Here's how the part is built. I have some questions about the finished solid (model axes, mm). A direction names the side the tool comes from. Coordinates: 2 decimals unless noted, no trailing zeros. Loops run counter-clockwise (first coordinate to the right, second up) from the corner with the lowest first, then second, coordinate; pieces in that order, holes last. Notation, with made-up numbers: M -5,31.25 L 54,31.25 A25 ccw 54,64.25 Z; hole C 31,54.5 d7. An arc over 180 degrees is marked long. Use CSV: the item, a comma, the result in double quotes. Start each with the question number.
Q1. Which directions (+Z, -Z, +X, -X, +Y, -Y) give clear straight access to the entire face, cutting with the end or side of a thin tool? Please do faces 4 (the cylindrical face through (-18.539, -3.905, -0.867)), 5 (the cylindrical face through (-14.985, 14.584, -0.66)).
Q2. Please list where these lines run through material, in increasing order: probe 1 along Z at (x, y) = (16, 0); probe 2 along X at (y, z) = (-18, 0). Write a range as [from, to].
Q3. For pin 1 Ø24 at (y, z) = (0, 0) entering from +X; pin 2 Ø1.5 at (y, z) = (-1, 7.5) entering from +X; pin 3 Ø7 at (x, z) = (0, 0) entering from -Y, each with a flat end and sliding along its axis, tell me the tip position at first contact or that it passes through.
Q4. If we section it at D-D (z = -11): Please give me the cut outline in (x, y).
Q5. If we section it at A-A (x = 0): Please give me the cut outline in (y, z), and give its area (3 significant figures).
Q6. If we section it at C-C (z = 0): Please give me the cut outline in (x, y).
Q7. If we mould it in two halves opening along Z, with no side actions, what happens to faces 1 (the cylindrical face through (-1.748, 18.859, -18.797)), 2 (the cylindrical face through (14.584, -14.643, 3.252)), 3 (the flat face through (-15.4, 20, -0.1))? For each: +Z half, -Z half, draft (parallel to the pull), parting line (faces both ways), or undercut.
from build123d import *

# Parameters (mm, degrees)
SKETCH1_W           = 40
SKETCH1_H           = 40
BOSS_EXTRUDE1_DEPTH = 20
FILLET1_R           = 4
SKETCH12_R          = 15
CUT_EXTRUDE2_DEPTH  = 20
SKETCH13_R          = 15
CUT_EXTRUDE3_DEPTH  = 20
SKETCH16_R          = 4
CUT_EXTRUDE6_DEPTH  = 20
SKETCH17_R          = 4
CUT_EXTRUDE7_DEPTH  = 20


with BuildPart() as part:
    # Sketch1 → Boss-Extrude1 (new body, symmetric)
    with BuildSketch(Plane(origin=(0, 0, 0), x_dir=(1, 0, 0), z_dir=(0, 1, 0))):
        Rectangle(SKETCH1_W, SKETCH1_H)
    extrude(amount=BOSS_EXTRUDE1_DEPTH, both=True)

    # Fillet1
    fillet1_edges = [part.edges().sort_by_distance(p)[0] for p in [
        (20, 20, 0),
        (0, 20, -20),
        (20, 0, -20),
        (20, 0, 20),
        (0, 20, 20),
    ]]
    fillet(fillet1_edges, radius=FILLET1_R)

    # Sketch2 → Cut-Revolve1 (revolve, cut)
    with BuildSketch(Plane(origin=(0, 0, 0), x_dir=(1, 0, 0), z_dir=(0, 1, 0))):
        with BuildLine():
            Line((0, 17.5), (0, -17.5))
            ThreePointArc((0, -17.5), (-17.5, 0), (0, 17.5))
        make_face()
    revolve(axis=Axis((0, 0, -20.989422068), (0, 0, 1)), mode=Mode.SUBTRACT)

    # Sketch12 → Cut-Extrude2 (cut)
    with BuildSketch(Plane(origin=(0, 20, 0), x_dir=(1, 0, 0), z_dir=(0, 1, 0))):
        Circle(SKETCH12_R)
    extrude(amount=-CUT_EXTRUDE2_DEPTH, mode=Mode.SUBTRACT)

    # Sketch13 → Cut-Extrude3 (cut)
    with BuildSketch(Plane(origin=(20, 0, 0), x_dir=(0, 0, -1), z_dir=(1, 0, 0))):
        Circle(SKETCH13_R)
    extrude(amount=-CUT_EXTRUDE3_DEPTH, mode=Mode.SUBTRACT)

    # Sketch16 → Cut-Extrude6 (cut)
    with BuildSketch(Plane.XZ.offset(20)):
        Circle(SKETCH16_R)
    extrude(amount=-CUT_EXTRUDE6_DEPTH, mode=Mode.SUBTRACT)

    # Sketch17 → Cut-Extrude7 (cut)
    with BuildSketch(Plane.ZY.offset(20)):
        Circle(SKETCH17_R)
    extrude(amount=-CUT_EXTRUDE7_DEPTH, mode=Mode.SUBTRACT)


solid = part.part
Results below:
1,face 4,"+X, -X"
1,face 5,"+Y"
2,probe 1,"[-20, -15], [15, 20]"
2,probe 2,"[-20, -4], [4, 20]"
3,pin 1,"x = -12.74"
3,pin 2,"x = -15.4"
3,pin 3,"through"
4,outline,"M -20,-20 L 20,-20 L 20,-10.2 L 9.01,-10.2 A13.61 cw -10.2,9.01 L -10.2,20 L -20,20 Z; M 10.2,10.2 L 20,10.2 L 20,16 A4 ccw 16,20 L 10.2,20 Z"
5,outline,"M -20,-20 L 16,-20 A4 ccw 20,-16 L 20,-15 L 9.01,-15 A17.5 cw -17.04,-4 L -20,-4 Z; M -20,4 L -17.04,4 A17.5 cw 9.01,15 L 20,15 L 20,16 A4 ccw 16,20 L -20,20 Z"
5,area,"460 mm^2"
6,outline,"M -20,-20 L -4,-20 L -4,-17.04 A17.5 cw -17.04,-4 L -20,-4 Z; M -20,4 L -17.04,4 A17.5 cw -15,9.01 L -15,20 L -20,20 Z; M 4,-20 L 20,-20 L 20,-15 L 9.01,-15 A17.5 cw 4,-17.04 Z; M 15,15 L 20,15 L 20,16 A4 ccw 16,20 L 15,20 Z"
7,face 1,"-Z half"
7,face 2,"undercut"
7,face 3,"draft"
